Work out the finished part from the listing and answer in its coordinate system (mm). Round coordinates to 2 decimals unless told otherwise and drop trailing zeros. Loops run counter-clockwise (first coordinate to the right, second up) from the corner with the lowest first, then second, coordinate; pieces in that order, holes last. Notation, with made-up numbers: (14, 65.5) - (35, 65.5) arc R15 ccw to (35, 74.5) - close; hole circle Ø5 at (76, 77.5). An arc over 180 degrees is marked (long way). Use CSV: the item, a comma, the result in double quotes. Start each with the question number.
from build123d import *

# Parameters (mm, degrees)
F0_R     = 22
F1_DEPTH = 0.5
F2_R     = 14.5
F3_DEPTH = 25
F5_DEPTH = 25


with BuildPart() as f1:
    # F0 (on Top) → F1 (new body)
    with BuildSketch(Plane.XY):
        Circle(F0_R)
    extrude(amount=F1_DEPTH)

    # F2 (on face) → F3 (cut)
    with BuildSketch(Plane.XY.offset(0.5)):
        Circle(F2_R)
    extrude(amount=-F3_DEPTH, mode=Mode.SUBTRACT)

    # F4 (on face) → F5 (cut)
    with BuildSketch(Plane.XY.offset(0.5)):
        with BuildLine():
            ThreePointArc((-1.0157200741, -21.9765400537), (0, -22), (1.0157200741, -21.9765400537))
            Line((1.0157200741, -21.9765400537), (1.0157200741, -14.4643808278))
            ThreePointArc((1.0157200741, -14.4643808278), (0, -14.5), (-1.0157200741, -14.4643808278))
            Line((-1.0157200741, -14.4643808278), (-1.0157200741, -21.9765400537))
        make_face()
    extrude(amount=-F5_DEPTH, mode=Mode.SUBTRACT)


solid = f1.part
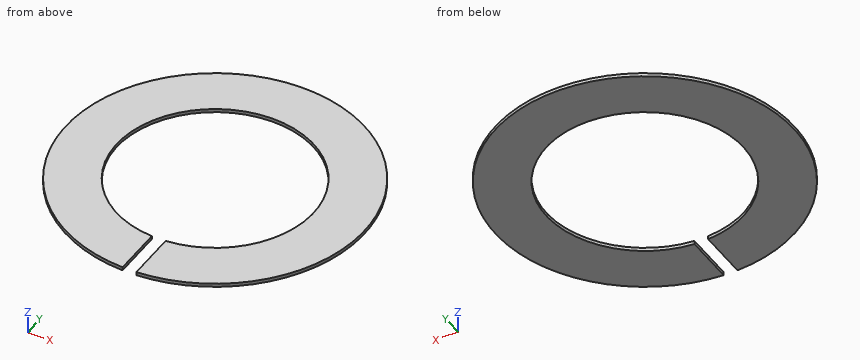
Item 1: A cutting plane is placed at B-B (x = -9). Determine the outline of the cut face in (y, z), plus the area to 3 significant figures.
Item 2: A cutting plane is placed at C-C (z = 0.25). Determine the outline of the cut face in (x, y), plus the area to 3 significant figures.
Item 3: A cutting plane is placed at D-D (x = 0). Determine the outline of the cut face in (y, z).
Item 4: Find the intervals of material crossed by probe 1 along X at (y, z) = (0, 0.25); probe 2 along Y at (x, z) = (9.5, 0.4); probe 3 along Y at (x, z) = (0, 0.35), in increasing order. Write a range as [from, to].
Item 5: A cutting plane is placed at A-A (y = 0). Determine the outline of the cut face in (x, z), plus the area to 3 significant figures.
Item 6: This flat-tipped pin is pushed along its axis until it touches: pin 1 Ø17.5 at (x, y) = (0, 0) entering from +Z. Where does it stop, or does it pass through?
Result sheet:
1,outline,"(-20.07, 0) - (-11.37, 0) - (-11.37, 0.5) - (-20.07, 0.5) - close; (11.37, 0) - (20.07, 0) - (20.07, 0.5) - (11.37, 0.5) - close"
1,area,"8.71 mm^2"
2,outline,"(-1.02, -21.98) - (-1.02, -14.46) arc R14.5 cw (long way) to (1.02, -14.46) - (1.02, -21.98) arc R22 ccw (long way) to start"
2,area,"845 mm^2"
3,outline,"(14.5, 0) - (22, 0) - (22, 0.5) - (14.5, 0.5) - close"
4,probe 1,"[-22, -14.5], [14.5, 22]"
4,probe 2,"[-19.84, -10.95], [10.95, 19.84]"
4,probe 3,"[14.5, 22]"
5,outline,"(-22, 0) - (-14.5, 0) - (-14.5, 0.5) - (-22, 0.5) - close; (14.5, 0) - (22, 0) - (22, 0.5) - (14.5, 0.5) - close"
5,area,"7.50 mm^2"
6,pin 1,"through"
